Here's how the part is built. I have some questions about the finished solid (model axes, mm). A direction names the side the tool comes from. Round coordinates to 2 decimals unless told otherwise and drop trailing zeros. Write each loop counter-clockwise with the first axis right and the second up, starting at its lowest first coordinate (ties: lowest second). Pieces come first, ordered by that corner, then holes. Notation, with made-up numbers: M 54,82.25 L 99,82.25 A28 ccw 99,107.25 Z; hole C -15,63 d8. An arc over 180 degrees is marked long. Write item = value, one per line. Start each with the question number.
(1) Will these pins go through, and if not, where does the flat tip stop? pin 1 Ø12.5 at (x, z) = (-68, 7) entering from +Y; pin 2 Ø12 at (y, z) = (5.5, 13.5) entering from +X; pin 3 Ø4 at (x, y) = (59, 2.5) entering from -Z; pin 4 Ø6.5 at (x, z) = (-96.5, 16.5) entering from -Y.
(2) If we mould it in two halves opening along X, with no side actions, what happens to faces 4 (the flat face through (-119.062, 11, 12)), 5 (the flat face through (-77.611, 6.726, 12.325)), 6 (the flat face through (-114, -16.734, 12))? For each: released by +X, released by -X, zero draft, split by the parting line, or undercut.
(3) On a 3-axis mill with a long thin cutter (end or side, diameter ignored), from which of +Z, -Z, +X, -X, +Y, -Y can I reach the whole of each face in a straight line? I mean faces 1 (the flat face through (15, 23, 0)), 2 (the flat face through (-40, 38.266, 12)), 3 (the flat face through (-104, 13.266, 12)). Say none if no direction works.
(4) I want a section at B-B (z = 14.75). List the corners of the cut face in (x, y) for me, and give its area (3 significant figures).
(5) I want a section at D-D (y = 2). List the corners of the cut face in (x, z) for me, and give its area (3 significant figures).
(6) I want a section at A-A (x = 78.5). List the corners of the cut face in (y, z) for me.
(7) I need wall thicknesses on line 1 along X through (y, z) = (6, 21); line 2 along X through (y, z) = (7.5, 2.5); line 3 along Y through (x, z) = (-66, 11.5). Which ranges of each line are inside material? Lowest first, please.
(8) I want a section at C-C (y = 23). List the corners of the cut face in (x, z) for me, and give its area (3 significant figures).
```python
from build123d import *

# Parameters (mm, degrees)
F0_R     = 17.5
F1_DEPTH = 25


with BuildPart() as f1:
    # F0 (on Top) → F1 (new body)
    with BuildSketch(Plane.XY):
        with BuildLine():
            Line((35.937557, 38.266499), (-119.062443, 38.266499))
            Line((-119.062443, 38.266499), (-119.062443, 13.266499))
            Line((-119.062443, 13.266499), (-119.062443, -16.733501))
            Line((-119.062443, -16.733501), (-109.062443, -16.733501))
            Line((-109.062443, -16.733501), (-109.062443, 13.266499))
            Line((-109.062443, 13.266499), (-99.062443, 13.266499))
            Line((-99.062443, 13.266499), (-99.062443, -1.733501))
            Line((-99.062443, -1.733501), (-91.062443, -1.733501))
            Line((-91.062443, -1.733501), (-91.062443, 13.266499))
            Line((-91.062443, 13.266499), (-81.062443, 13.266499))
            Line((-81.062443, 13.266499), (-74.062443, 0))
            Line((-74.062443, 0), (-67.062443, 13.266499))
            Line((-67.062443, 13.266499), (35.937557, 13.266499))
            ThreePointArc((35.937557, 13.266499), (103.629299, 25.766499), (35.937557, 38.266499))
        make_face()
        with Locations((68.629299, 25.766499)):
            Circle(F0_R, mode=Mode.SUBTRACT)
    extrude(amount=F1_DEPTH)


solid = f1.part
```
Returned:
q1.pin_1 = 38.27
q1.pin_2 = 100.59
q1.pin_3 = 0
q1.pin_4 = -1.73
q2.face_4 = released by -X
q2.face_5 = undercut
q2.face_6 = zero draft
q3.face_1 = -Z, +X, -X, +Y, -Y
q3.face_2 = +Z, -Z, -X, +Y
q3.face_3 = +Z, -Z, -Y
q4.outline = M -119.06,-16.73 L -109.06,-16.73 L -109.06,13.27 L -99.06,13.27 L -99.06,-1.73 L -91.06,-1.73 L -91.06,13.27 L -81.06,13.27 L -74.06,0 L -67.06,13.27 L 35.94,13.27 A35 ccw long 35.94,38.27 L -119.06,38.27 Z; hole C 68.63,25.77 d35
q4.area = 7,240 mm²
q5.outline = M -119.06,0 L -109.06,0 L -109.06,25 L -119.06,25 Z; M -99.06,0 L -91.06,0 L -91.06,25 L -99.06,25 Z; M -75.12,0 L -73.01,0 L -73.01,25 L -75.12,25 Z; M 42.94,0 L 94.32,0 L 94.32,25 L 42.94,25 Z
q5.area = 1,790 mm²
q6.outline = M -7.81,0 L 11.32,0 L 11.32,25 L -7.81,25 Z; M 40.22,0 L 59.35,0 L 59.35,25 L 40.22,25 Z
q7.line_1 = -119.06 to -109.06, -99.06 to -91.06, -77.23 to -70.9, 39.75 to 97.51
q7.line_2 = -119.06 to -109.06, -99.06 to -91.06, -78.02 to -70.11, 38.77 to 98.48
q7.line_3 = 13.27 to 38.27
q8.outline = M -119.06,0 L 51.35,0 L 51.35,25 L -119.06,25 Z; M 85.91,0 L 103.52,0 L 103.52,25 L 85.91,25 Z
q8.area = 4,700 mm²
